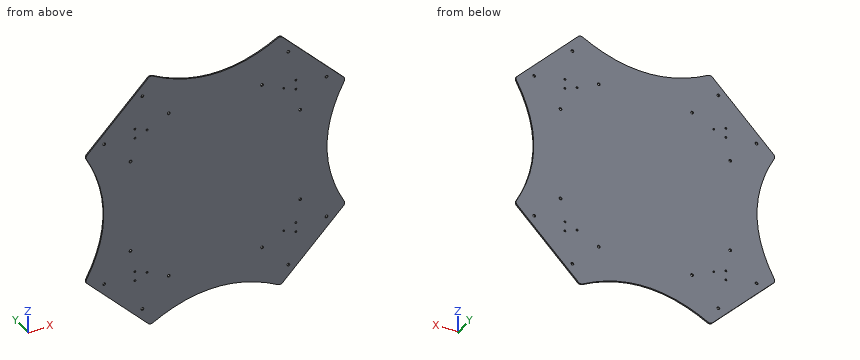
```python
from build123d import *

# Parameters (mm, degrees)
DODANIE_WYCI_GNI_CIE1_DEPTH = 1.5
ZAOKR_GLENIE1_R             = 4
SZKIC2_R                    = 1.5
WYTNIJ_WYCI_GNI_CIE1_DEPTH  = 197.62293997
SZYK_KO_OWY1_COUNT          = 4
SZKIC3_R                    = 1
WYTNIJ_WYCI_GNI_CIE2_DEPTH  = 197.62293997
SZYK_KO_OWY2_OUTLINE_R      = 1
SZYK_KO_OWY2_DEPTH          = 1.5


# Read off the part's stored shape, not the designer's step: Szyk kołowy2
with BuildPart() as part:
    # Szkic1 → Dodanie-wyciągnięcie1 (new body)
    with BuildSketch(Plane(origin=(0, 0, 0), x_dir=(1, 0, 0), z_dir=(0, 1, 0))):
        with BuildLine():
            Line((-70, -140), (-140, -70))
            add(Edge.make_bspline(
                [(-140, 70), (-100, 0), (-140, -70)],
                knots=[0, 0, 0, 1, 1, 1], degree=2))
            Line((-140, 70), (-70, 140))
            add(Edge.make_bspline(
                [(70, 140), (0, 100), (-70, 140)],
                knots=[0, 0, 0, 1, 1, 1], degree=2))
            Line((70, 140), (140, 70))
            add(Edge.make_bspline(
                [(140, -70), (100, 0), (140, 70)],
                knots=[0, 0, 0, 1, 1, 1], degree=2))
            Line((140, -70), (70, -140))
            add(Edge.make_bspline(
                [(-70, -140), (0, -100), (70, -140)],
                knots=[0, 0, 0, 1, 1, 1], degree=2))
        make_face()
    extrude(amount=DODANIE_WYCI_GNI_CIE1_DEPTH)

    # Zaokrąglenie1
    zaokr_glenie1_edges = [part.edges().sort_by_distance(p)[0] for p in [
        (-140, 0.75, -70),
        (-70, 0.75, -140),
        (70, 0.75, -140),
        (140, 0.75, -70),
        (140, 0.75, 70),
        (70, 0.75, 140),
        (-140, 0.75, 70),
        (-70, 0.75, 140),
    ]]
    fillet(zaokr_glenie1_edges, radius=ZAOKR_GLENIE1_R)

    # Szkic2 → Wytnij-wyciągnięcie1 (cut, through all)
    with BuildSketch(Plane(origin=(0, 1.5, 0), x_dir=(1, 0, 0), z_dir=(0, 1, 0))):
        with Locations(Location((-78.488852712, -119.501046021, 0), (0, 0, 270))):
            Circle(SZKIC2_R)
        with Locations(Location((-119.501046021, -78.488852712, 0), (0, 0, 90))):
            Circle(SZKIC2_R)
        with Locations(Location((-50.204581464, -91.216774773, 0), (0, 0, 90))):
            Circle(SZKIC2_R)
        with Locations(Location((-91.216774773, -50.204581464, 0), (0, 0, 270))):
            Circle(SZKIC2_R)
    wytnij_wyci_gni_cie1 = extrude(amount=-WYTNIJ_WYCI_GNI_CIE1_DEPTH, mode=Mode.SUBTRACT)

    # Szyk kołowy1: Wytnij-wyciągnięcie1 ×4 about axis
    szyk_ko_owy1_axis = Axis((0, 0, 0), (0, 1, 0))
    for i in range(1, SZYK_KO_OWY1_COUNT):
        add(wytnij_wyci_gni_cie1.rotate(szyk_ko_owy1_axis, i * 360 / SZYK_KO_OWY1_COUNT), mode=Mode.SUBTRACT)

    # Szkic3 → Wytnij-wyciągnięcie2 (cut, through all)
    with BuildSketch(Plane(origin=(0, 1.5, 0), x_dir=(1, 0, 0), z_dir=(0, 1, 0))):
        with Locations(Location((-86.525, -85.085, 0), (0, 0, 270))):
            Circle(SZKIC3_R)
        with Locations(Location((-73.475, -80, 0), (0, 0, 270))):
            Circle(SZKIC3_R)
        with Locations(Location((-86.525, -74.915, 0), (0, 0, 90))):
            Circle(SZKIC3_R)
    wytnij_wyci_gni_cie2 = extrude(amount=-WYTNIJ_WYCI_GNI_CIE2_DEPTH, mode=Mode.SUBTRACT)

    # Lustro1: Wytnij-wyciągnięcie2 across plane
    add(wytnij_wyci_gni_cie2.mirror(Plane(origin=(0, 0, 0), x_dir=(0, 0, 1), z_dir=(1, 0, 0))), mode=Mode.SUBTRACT)

    # Szyk kołowy2 outline → Szyk kołowy2 (cut)
    with BuildSketch(Plane(origin=(0, 0, 0), x_dir=(1, 0, 0), z_dir=(0, 1, 0))):
        with Locations((-86.525, 74.915)):
            Circle(SZYK_KO_OWY2_OUTLINE_R)
        with Locations((-73.475, 80)):
            Circle(SZYK_KO_OWY2_OUTLINE_R)
        with Locations((-86.525, 85.085)):
            Circle(SZYK_KO_OWY2_OUTLINE_R)
        with Locations((86.525, 85.085)):
            Circle(SZYK_KO_OWY2_OUTLINE_R)
        with Locations((86.525, 74.915)):
            Circle(SZYK_KO_OWY2_OUTLINE_R)
        with Locations((73.475, 80)):
            Circle(SZYK_KO_OWY2_OUTLINE_R)
    extrude(amount=SZYK_KO_OWY2_DEPTH, mode=Mode.SUBTRACT)


solid = part.part
```
Check sheet for the modelled part. Datum: model origin and axes. Units: mm. Coordinates: 2 decimals unless noted, no trailing zeros. Order: outer loops, then holes, each group sorted by start corner. A loop starts at its lowest first (then second) coordinate and runs counter-clockwise, first axis right, second up. Notation, with made-up numbers: M 77.25,-4 L 132.25,-4 A24 ccw 132.25,12 Z; hole C -5,38 d7. An arc over 180 degrees is marked long. One line per question, with ' | ' between items. Start each with the question number.
Item 1: Sectioned sample at C-C on z = 96.5. Record the cut outline in (x, y).
Item 2: Sectioned sample at A-A on x = -108.5. Record the cut outline in (y, z).
Item 3: Sectioned sample at B-B on y = 1.2. Count the separate pieces of the cut face and the enclosed holes in it, and give its area (3 significant figures).
Item 4: Material ranges on line 1 (Z direction, x = -91.5, y = 0.75); line 2 (X direction, y = 1, z = 78.5); line 3 (X direction, y = 0.6, z = -15), recorded low to high.
Item 5: Gauge pin test, flat end, axial feed: P1, Ø1.8, axis at x = -86.525, z = 85.085, coming from the -Y side. Record the tip position at first contact, or that the pin passes through.
Answer below:
1) outline: M -113.5,0 L 113.5,0 L 113.5,1.5 L -113.5,1.5 Z
2) outline: M 0,-101.5 L 1.5,-101.5 L 1.5,101.5 L 0,101.5 Z
3) separate pieces: 1 | enclosed holes: 28 | area: 61,000 mm^2
4) line 1: z = -118.5 to -51.68, -48.73 to 48.73, 51.68 to 118.5 | line 2: x = -131.5 to -121, -118 to 118, 121 to 131.5 | line 3: x = -120.92 to 120.92
5) P1: passes through
